Could you check a few things on this drawing? It's one solid part, dimensions in mm from its lowest x, y, z. Give positions to 0.01 mm unless a question says otherwise; leave off trailing zeros. Order: outer loops, then holes, each group sorted by start corner. A loop starts at its lowest first (then second) coordinate and runs counter-clockwise, first axis right, second up.
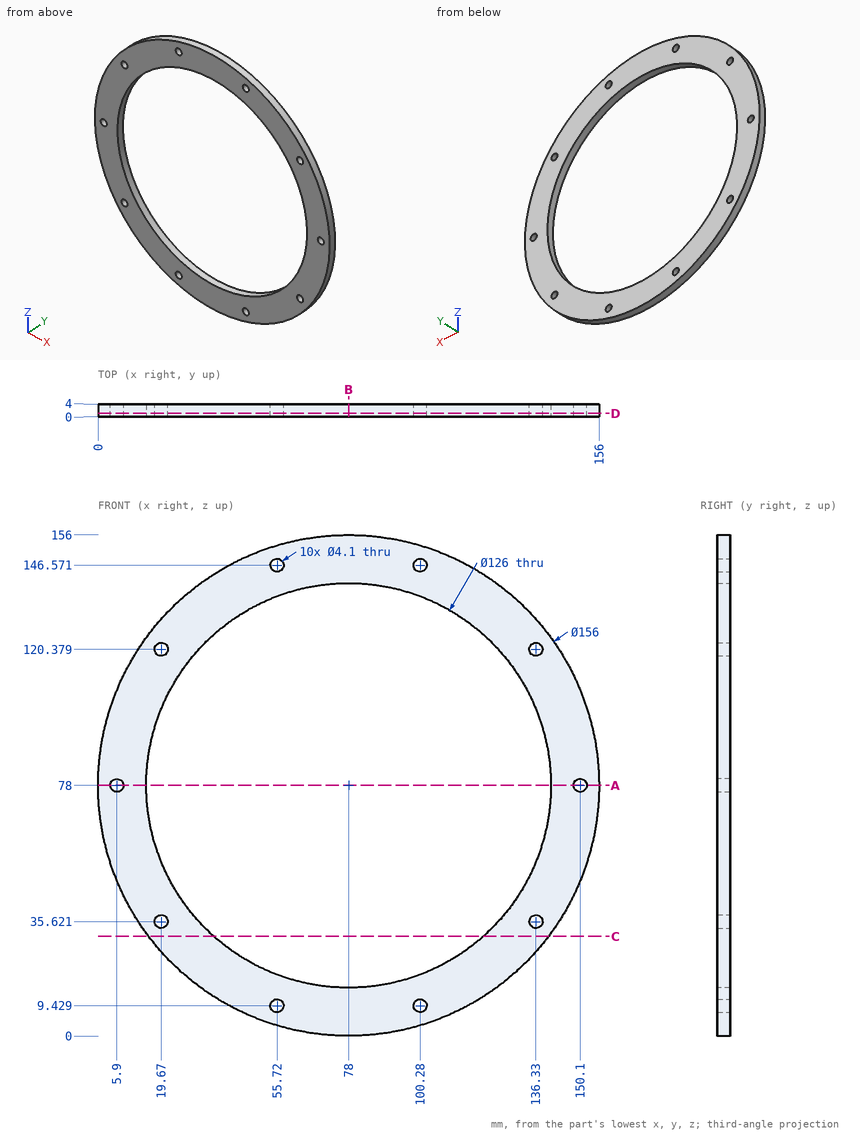
Item 1: Imagine slicing it at B-B on x = 78. List the corners of the cut face in (y, z) for me.
Findings:
outline: (0, 0) - (4, 0) - (4, 15) - (0, 15) - close; (0, 141) - (4, 141) - (4, 156) - (0, 156) - close
Item 2: Please list where these lines run through material, in increasing order: line 1 along X through (y, z) = (0.75, 11) (1 decimal); line 2 along Z through (x, y) = (56, 3.7); line 3 along X through (y, z) = (1.15, 78).
Findings:
line 1: x = 38.1 to 54.4, 57 to 99, 101.6 to 117.9
line 2: z = 3.17 to 7.4, 11.46 to 18.97, 137.03 to 144.54, 148.6 to 152.83
line 3: x = 0 to 3.85, 7.95 to 15, 141 to 148.05, 152.15 to 156
Item 3: For pin 1 (3.5 mm diameter, centred on x = 55.72, z = 146.57, fed in from +Y); pin 2 (5.5 mm diameter, centred on x = 5.9, z = 78, fed in from -Y); pin 3 (2 mm diameter, centred on x = 69, y = 1, fed in from -Z), each with a flat end and sliding along its axis, tell me the tip position at first contact or that it passes through.
Findings:
pin 1: passes through
pin 2: stops at y = 0
pin 3: stops at z = 0.41
Item 4: Imagine slicing it at D-D on y = 1.05. Give the number of separate pieces and of enclosed holes in the cut face, then the cut area to 3 significant figures.
Findings:
separate pieces: 1
enclosed holes: 11
area: 6,510 mm2
Item 5: Imagine slicing it at C-C on z = 31. List the corners of the cut face in (x, y) for me.
Findings:
outline: (15.75, 0) - (36.05, 0) - (36.05, 4) - (15.75, 4) - close; (119.95, 0) - (140.25, 0) - (140.25, 4) - (119.95, 4) - close
Item 6: Imagine slicing it at A-A on z = 78. List the corners of the cut face in (x, y) for me, then the cut area to 3 significant figures.
Findings:
outline: (0, 0) - (3.85, 0) - (3.85, 4) - (0, 4) - close; (7.95, 0) - (15, 0) - (15, 4) - (7.95, 4) - close; (141, 0) - (148.05, 0) - (148.05, 4) - (141, 4) - close; (152.15, 0) - (156, 0) - (156, 4) - (152.15, 4) - close
area: 87.2 mm2
